from build123d import *

# Parameters (mm, degrees)
SKETCH1_R           = 47.625
SKETCH1_R_2         = 3.3
BOSS_EXTRUDE1_DEPTH = 4.7625
SKETCH4_R           = 3.3
CUT_EXTRUDE2_DEPTH  = 10.525


with BuildPart() as part:
    # Sketch1 → Boss-Extrude1 (new body, symmetric)
    with BuildSketch(Plane(origin=(0, 0, 0), x_dir=(1, 0, 0), z_dir=(0, 1, 0))):
        Circle(SKETCH1_R)
        Circle(SKETCH1_R_2, mode=Mode.SUBTRACT)
    extrude(amount=BOSS_EXTRUDE1_DEPTH, both=True)

    # Sketch4 → Cut-Extrude2 (cut, through all)
    with BuildSketch(Plane(origin=(0, 4.7625, 0), x_dir=(1, 0, 0), z_dir=(0, 1, 0))):
        with Locations((-12.900657786, -35.444265963)):
            Circle(SKETCH4_R)
        with Locations((-24.24530585, 28.89443035)):
            Circle(SKETCH4_R)
        with Locations((37.145963636, 6.549835613)):
            Circle(SKETCH4_R)
        with Locations((14.285954625, -17.025337748)):
            Circle(SKETCH4_R)
        with Locations((-21.887352311, -3.859330749)):
            Circle(SKETCH4_R)
        with Locations((7.601397685, 20.884668497)):
            Circle(SKETCH4_R)
    extrude(amount=-CUT_EXTRUDE2_DEPTH, mode=Mode.SUBTRACT)


solid = part.part
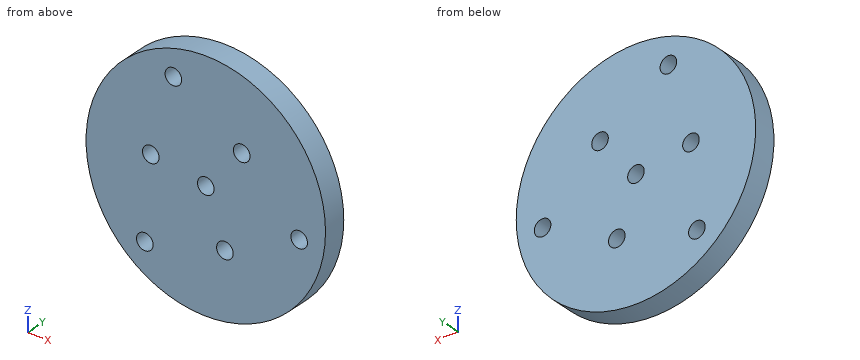
Input: part model. Units: mm. Frame: model coordinates. Round coordinates to 2 decimals unless told otherwise and drop trailing zeros. Write each loop counter-clockwise with the first axis right and the second up, starting at its lowest first coordinate (ties: lowest second). Pieces come first, ordered by that corner, then holes.
1) Cut plane C-C (y = 1). Return the cut outline in (x, z) (3 decimals), then the cut area to 3 significant figures.
2) Cut plane A-A (x = 0). Return the cut outline in (y, z) (1 decimal).
3) Contact query for flat-ended pins moving along their axis: P1, Ø6, axis at x = -21.89, z = 3.86, coming from the -Y side; P2, Ø1, axis at x = -15.5, y = -1, coming from the +Z side; P3, Ø2, axis at y = 1, z = 32.5, coming from the -X side; P4, Ø7.5, axis at x = 0, z = 0, coming from the +Y side. Output: stop coordinate, or through.
4) Cut plane D-D (z = 40.5). Return the cut outline in (x, y).
5) Ray query, L1, parallel to X at y = 3.75, z = 18.5; L2, parallel to X at y = -2, z = 19; L3, parallel to Z at x = -11.5, y = -3.75. Return the intervals inside material, ascending.
6) Cut plane B-B (z = 6). Return the cut outline in (x, y), then the cut area to 3 significant figures.
Geometry says:
1. outline: circle Ø95.25 at (0, 0); hole circle Ø6.6 at (-24.245, -28.894); hole circle Ø6.6 at (-21.887, 3.859); hole circle Ø6.6 at (-12.901, 35.444); hole circle Ø6.6 at (0, 0); hole circle Ø6.6 at (7.601, -20.885); hole circle Ø6.6 at (14.286, 17.025); hole circle Ø6.6 at (37.146, -6.55)
1. area: 6,890 mm2
2. outline: (-4.8, -47.6) - (4.8, -47.6) - (4.8, -3.3) - (-4.8, -3.3) - close; (-4.8, 3.3) - (4.8, 3.3) - (4.8, 47.6) - (-4.8, 47.6) - close
3. P1: passes through
3. P2: stops at z = 45.2
3. P3: stops at x = -35.72
3. P4: stops at y = 4.76
4. outline: (-25.06, -4.76) - (25.06, -4.76) - (25.06, 4.76) - (-25.06, 4.76) - close
5. L1: x = -43.88 to 11.33, 17.24 to 43.88
5. L2: x = -43.67 to 11.64, 16.93 to 43.67
5. L3: z = -46.22 to 32.46, 38.43 to 46.22
6. outline: (-47.25, -4.76) - (-24.4, -4.76) - (-24.4, 4.76) - (-47.25, 4.76) - close; (-19.38, -4.76) - (47.25, -4.76) - (47.25, 4.76) - (-19.38, 4.76) - close
6. area: 852 mm2
